```python
from build123d import *

# Parameters (mm, degrees)
F2_DEPTH      = 165.1
F2_DEPTH_BACK = 165.1
F3_DEPTH      = 13.2243322
F0_W          = 297.7512968
F0_H          = 107.2502808
F0_W_2        = 287.2877414
F0_H_2        = 96.8048356
F4_DEPTH      = 11.43


with BuildPart() as f2:
    # F1 (on Right) → F2 (new body, two sides)
    with BuildSketch(Plane.YZ) as f2_sk:
        Polygon((0, -69.85), (0, 0), (0, 69.85), (-12.12932521, -68.7888215479), align=None)
    extrude(amount=F2_DEPTH)
    extrude(f2_sk.sketch, amount=-F2_DEPTH_BACK)

    # F3 (add): a face of the model
    f3_faces = [f2.faces().sort_by_distance(p)[0] for p in [
        (0, -6.064662605, 0.530589226),
    ]]
    extrude(f3_faces, amount=F3_DEPTH)

    # F0 (on Front) → F4 (cut)
    with BuildSketch(Plane.XZ):
        Rectangle(F0_W, F0_H)
        Rectangle(F0_W_2, F0_H_2, mode=Mode.SUBTRACT)
        Rectangle(F0_W_2, F0_H_2)
    extrude(amount=F4_DEPTH, mode=Mode.SUBTRACT)


solid = f2.part
```
Part model, mm, in its own coordinate system. A direction names the side the tool comes from. Round coordinates to 2 decimals unless told otherwise and drop trailing zeros. Write each loop counter-clockwise with the first axis right and the second up, starting at its lowest first coordinate (ties: lowest second). Pieces come first, ordered by that corner, then holes. Notation, with made-up numbers: M 27.25,-38.5 L 50.25,-38.5 A9 cw 50.25,-28.5 Z; hole C 26.5,45.5 d7. An arc over 180 degrees is marked long. Answer as CSV lines item,"result". Start each with the question number.
1) Mould opens along Z. For faces 3 (the face through (13, 0, -57)), 4 (the face through (148.876, -6, -1)), 5 (the face through (2.311, -19.154, 2.654)) say: +Z half, -Z half, draft (parallel to the pull), parting line (faces both ways), or undercut.
2) Which spindle directions (+Z, -Z, +X, -X, +Y, -Y) get a long thin tool onto all of the face, cutting with end or side? Do faces 1 (the face through (-165.1, -9, 2)), 2 (the face through (-2, -11.43, 1)). Say none if no direction does.
3) Drop flat-ended pins along their axis: pin 1 (3.5 mm diameter, centred on x = 61, y = -5.5, fed in from -Z); pin 2 (2 mm diameter, centred on x = -86, y = -5, fed in from +Z); pin 3 (10 mm diameter, centred on x = -6.5, y = -16.5, fed in from -Z). Give the stop position or say it passes through.
4) Drill centre lines: L1, parallel to X at y = -10.5, z = -13; L2, parallel to Z at x = -129, y = -4.5; L3, parallel to Z at x = 92, y = -6.5. Where is each one in solid material? Low to high.
5) Band-saw the part on B-B (x = 6). List the corners of the cut face in (y, z), then the cut area to 3 significant figures.
6) Band-saw the part on D-D (y = -19.75). List the corners of the cut face in (x, z), then the cut area to 3 significant figures.
7) Band-saw the part on C-C (z = -42.5). List the corners of the cut face in (x, y).
8) Band-saw the part on A-A (y = -3). List the corners of the cut face in (x, z).
Worked out:
1,face 3,"draft"
1,face 4,"undercut"
1,face 5,"+Z half"
2,face 1,"+Z, -Z, -X, +Y, -Y"
2,face 2,"+Y"
3,pin 1,"z = -69.52"
3,pin 2,"z = 70.37"
3,pin 3,"z = -68.84"
4,L1,"-165.1 to -148.88, 148.88 to 165.1"
4,L2,"-69.46 to -53.63, 53.63 to 70.24"
4,L3,"-69.28 to -53.63, 53.63 to 70.42"
5,outline,"M -25.3,-67.64 L 0,-69.85 L 0,-53.63 L -11.43,-53.63 L -11.43,53.63 L 0,53.63 L 0,69.85 L -13.17,71 Z"
5,area,"1,460 mm²"
6,outline,"M -165.1,-68.12 L 165.1,-68.12 L 165.1,-4.16 L -165.1,-4.16 Z"
6,area,"21,100 mm²"
7,outline,"M -165.1,-23.1 L 165.1,-23.1 L 165.1,0 L 148.88,0 L 148.88,-11.43 L -148.88,-11.43 L -148.88,0 L -165.1,0 Z"
8,outline,"M -165.1,-69.59 L 165.1,-69.59 L 165.1,70.11 L -165.1,70.11 Z; hole M -148.88,-53.63 L 148.88,-53.63 L 148.88,53.63 L -148.88,53.63 Z"
